Source: CAD feature listing. Evaluate the final solid. Frame: model axes, mm. A direction names the side the tool comes from. Coordinates: 2 decimals unless noted, no trailing zeros. Loops run counter-clockwise (first coordinate to the right, second up) from the corner with the lowest first, then second, coordinate; pieces in that order, holes last. Notation, with made-up numbers: (-27.5, 88.5) - (30.5, 88.5) arc R26 ccw to (30.5, 125.5) - close; hole circle Ø1 at (-18, 21). An arc over 180 degrees is marked (long way). Write item = value, one per line. Start each with the question number.
from build123d import *

# Parameters (mm, degrees)
F1_DEPTH = 20
F2_R     = 10.75
F3_DEPTH = 5
F4_R     = 10.75
F5_DEPTH = 5
F6_R     = 3.175
F7_DEPTH = 5
F8_R     = 3.175
F9_DEPTH = 5


with BuildPart() as f1:
    # F0 (on Front) → F1 (new body)
    with BuildSketch(Plane.XZ):
        with BuildLine():
            Line((37.5, -3.077656), (37.5, 1.988685))
            ThreePointArc((37.5, 1.988685), (0, 5), (-37.5, 1.988685))
            Line((-37.5, 1.988685), (-37.5, -3.077656))
            ThreePointArc((-37.5, -3.077656), (0, 0), (37.5, -3.077656))
        make_face()
    extrude(amount=F1_DEPTH)

    # F2 (on face) → F3 (join)
    with BuildSketch(Plane.YZ.offset(37.5)):
        with BuildLine():
            Line((0, 1.988685), (27.749921, 31.642143))
            ThreePointArc((27.749921, 31.642143), (25.071711, 55.451453), (1.978662, 49.066537))
            Line((1.978662, 49.066537), (-20, 1.988685))
            Line((-20, 1.988685), (0, 1.988685))
        make_face()
        with Locations((16.250001, 42.403851)):
            Circle(F2_R, mode=Mode.SUBTRACT)
    extrude(amount=-F3_DEPTH)

    # F4 (on face) → F5 (join)
    with BuildSketch(Plane(origin=(-37.5, 0, 0), x_dir=(0, -1, 0), z_dir=(-1, 0, 0))):
        with BuildLine():
            Line((20, 1.988685), (-1.978662, 49.066537))
            ThreePointArc((-1.978662, 49.066537), (-25.071711, 55.451453), (-27.749921, 31.642143))
            Line((-27.749921, 31.642143), (0, 1.988685))
            Line((0, 1.988685), (20, 1.988685))
        make_face()
        with Locations((-16.250001, 42.403851)):
            Circle(F4_R, mode=Mode.SUBTRACT)
    extrude(amount=-F5_DEPTH)

    # F6 (on face) → F7 (join)
    with BuildSketch(Plane.YZ.offset(37.5)):
        Polygon((0, 1.988685), (0, -3.077656), (12.772466, -3.077656), (12.772466, 15.637293), align=None)
        with Locations((7.242475, 2.498732)):
            Circle(F6_R, mode=Mode.SUBTRACT)
    extrude(amount=-F7_DEPTH)

    # F8 (on face) → F9 (join)
    with BuildSketch(Plane(origin=(-37.5, 0, 0), x_dir=(0, -1, 0), z_dir=(-1, 0, 0))):
        Polygon((-12.822957, -3.077656), (0, -3.077656), (0, 1.988685), (-12.822957, 15.691247), align=None)
        with Locations((-7.242475, 2.498732)):
            Circle(F8_R, mode=Mode.SUBTRACT)
    extrude(amount=-F9_DEPTH)


solid = f1.part
Item 1: Material intervals for L1, parallel to X at y = 9.5, z = 13; L2, parallel to Z at x = 33, y = 24 (3 decimals); L3, parallel to Z at x = -11.5, y = -5.5, sorted ascending. Write a range as [from, to].
Item 2: Cut plane B-B (z = 21.5). Return the cut outline in (x, y).
Item 3: Cut plane C-C (z = 51). Return the cut outline in (x, y), then the cut area to 3 significant figures.
Item 4: First-contact query: pin 1 (2.5 mm diameter, centred on x = -35, z = 4, fed in from +Y); pin 2 (4 mm diameter, centred on y = 7.24, z = 2.5, fed in from +X); pin 3 (3.5 mm diameter, centred on x = -11.5, z = 2.5, fed in from +Y). Flat tips, straight axial feed; report the tip coordinate or a pass-through.
Item 5: Cut plane D-D (y = -5). Return the cut outline in (x, z).
Item 6: Reachability of faces 5 (the flat face through (35, 6, -3.078)), 6 (the flat face through (-35, 12.823, 6)) from +Z, -Z, +X, -X, +Y, -Y: full face, straight path, thin tool, end or side. Return the list, or none.
Item 7: Draft query along Z for faces 1 (the flat face through (-35.035, -9.165, 25.198)), 2 (the cylindrical face through (35.035, 14.851, 53.062)), 3 (the flat face through (-1, -20, 2)), 4 (the cylindrical face through (-0.5, -9.9, 0)). Return one class per face: released by +Z, released by -Z, zero draft, split by the parting line, or undercut.
Item 8: Cut plane A-A (y = 14). Return the cut outline in (x, z).
Responses:
q1.L1 = [-37.5, -32.5], [32.5, 37.5]
q1.L2 = [27.635, 34.954], [49.854, 56.115]
q1.L3 = [-0.29, 4.72]
q2.outline = (-37.5, -10.89) - (-32.5, -10.89) - (-32.5, 18.26) - (-37.5, 18.26) - close; (32.5, -10.89) - (37.5, -10.89) - (37.5, 18.26) - (32.5, 18.26) - close
q3.outline = (-37.5, 3.05) - (-32.5, 3.05) - (-32.5, 9.79) - (-37.5, 9.79) - close; (-37.5, 22.71) - (-32.5, 22.71) - (-32.5, 29.45) - (-37.5, 29.45) - close; (32.5, 3.05) - (37.5, 3.05) - (37.5, 9.79) - (32.5, 9.79) - close; (32.5, 22.71) - (37.5, 22.71) - (37.5, 29.45) - (32.5, 29.45) - close
q3.area = 135 mm2
q4.pin_1 = 12.82
q4.pin_2 = through
q4.pin_3 = 0
q5.outline = (-37.5, -3.08) arc R230 cw to (37.5, -3.08) - (37.5, 34.12) - (32.5, 34.12) - (32.5, 2.74) arc R235 ccw to (-32.5, 2.74) - (-32.5, 34.12) - (-37.5, 34.12) - close
q6.face_5 = -Z, +X, -X, +Y, -Y
q6.face_6 = -Z, +X, -X, +Y
q7.face_1 = released by +Z
q7.face_2 = undercut
q7.face_3 = zero draft
q7.face_4 = released by -Z
q8.outline = (-37.5, 16.95) - (-32.5, 16.95) - (-32.5, 31.89) - (-37.5, 31.89) - close; (-37.5, 52.92) - (-32.5, 52.92) - (-32.5, 57.99) - (-37.5, 57.99) - close; (32.5, 16.95) - (37.5, 16.95) - (37.5, 31.89) - (32.5, 31.89) - close; (32.5, 52.92) - (37.5, 52.92) - (37.5, 57.99) - (32.5, 57.99) - close
